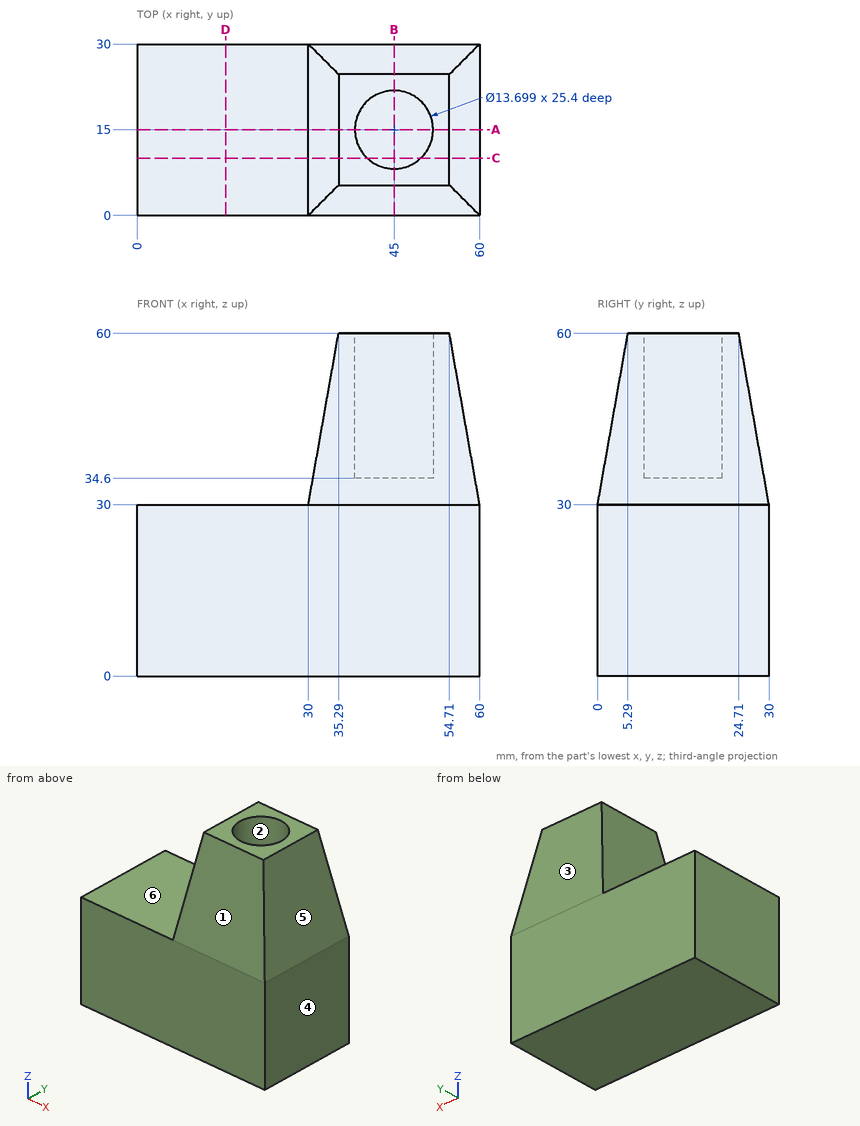
Could you check a few things on this drawing? It's one solid part, dimensions in mm from its lowest x, y, z. A direction names the side the tool comes from. Round coordinates to 2 decimals unless told otherwise and drop trailing zeros. Write each loop counter-clockwise with the first axis right and the second up, starting at its lowest first coordinate (ties: lowest second). Pieces come first, ordered by that corner, then holes.
Q1. Will these pins go through, and if not, where does the flat tip stop? P1, Ø3, axis at x = 41, z = 36, coming from the -Y side; P2, Ø5, axis at y = 7, z = 7, coming from the -X side; P3, Ø10, axis at y = 16, z = 36, coming from the -X side; P4, Ø9, axis at x = 17, y = 15, coming from the +Z side.
Q2. If we section it at A-A on y = 15: Write out the boundary of the cut face in (x, z), plus the area to 3 significant figures.
Q3. Please list where these lines run through material, in increasing order: probe 1 along Z at (x, y) = (12.5, 12); probe 2 along Y at (x, z) = (45, 51); probe 3 along Z at (x, y) = (42, 18).
Q4. If we section it at B-B on x = 45: Write out the boundary of the cut face in (y, z).
Q5. If we section it at C-C on y = 10: Write out the boundary of the cut face in (x, z).
Q6. Which directions (+Z, -Z, +X, -X, +Y, -Y) give clear straight access to the entire face, cutting with the end or side of a thin tool? Please do the marked faces 5 and 6.
Q7. If we section it at D-D on x = 15.5: Write out the boundary of the cut face in (y, z).
Q8. If we mould it in two halves opening along Y, with no side actions, what happens to the marked faces 1, 2, 3 and 4? For each: +Y half, -Y half, draft (parallel to the pull), parting line (faces both ways), or undercut.
Answer below:
1. P1: stops at y = 0.79
1. P2: stops at x = 0
1. P3: stops at x = 30.18
1. P4: stops at z = 30
2. outline: (0, 0) - (60, 0) - (60, 30) - (54.71, 60) - (51.85, 60) - (51.85, 34.6) - (38.15, 34.6) - (38.15, 60) - (35.29, 60) - (30, 30) - (0, 30) - close
2. area: 2,190 mm2
3. probe 1: z = 0 to 30
3. probe 2: y = 3.7 to 8.15, 21.85 to 26.3
3. probe 3: z = 0 to 34.6
4. outline: (0, 0) - (30, 0) - (30, 30) - (24.71, 60) - (21.85, 60) - (21.85, 34.6) - (8.15, 34.6) - (8.15, 60) - (5.29, 60) - (0, 30) - close
5. outline: (0, 0) - (60, 0) - (60, 30) - (54.71, 60) - (49.68, 60) - (49.68, 34.6) - (40.32, 34.6) - (40.32, 60) - (35.29, 60) - (30, 30) - (0, 30) - close
6. face 5: +Z, +X, +Y, -Y
6. face 6: +Z, -X, +Y, -Y
7. outline: (0, 0) - (30, 0) - (30, 30) - (0, 30) - close
8. face 1: -Y half
8. face 2: undercut
8. face 3: +Y half
8. face 4: draft
